The figure shows three views and two pictorial views of one solid part (mm, origin at its lowest corner). Answer the questions. A direction names the side the tool comes from. Round coordinates to 2 decimals unless told otherwise and drop trailing zeros. Order: outer loops, then holes, each group sorted by start corner. A loop starts at its lowest first (then second) coordinate and runs counter-clockwise, first axis right, second up. Notation, with made-up numbers: (30.5, 62.5) -> (88.5, 62.5) arc R19 ccw to (88.5, 91.5) -> close; hole circle Ø11 at (13, -25.75). An arc over 180 degrees is marked (long way). Answer as a JSON object with one key per item and string values. Group by question number.
Item 1: Given P1, Ø4, axis at x = 33.5, y = 25, coming from the +Z side; P2, Ø1, axis at x = 17, y = 8, coming from the -Z side; P3, Ø5.5, axis at x = 11.5, y = 24, coming from the +Z side (1 decimal), each flat-ended and moving along its own axis, determine where each tip first touches the part or whether it passes through.
Item 2: The mould has two halves that part along Z. Classify the marked faces 4, 5, 6 and 7: pulls with the +Z half, pulls with the -Z half, needs draft (parallel to the pull), parting line crosses it, or undercut.
Item 3: Section C-C, the plane y = 22.5 is taken. Write down the section's boundary in (x, z).
Item 4: Section A-A, the plane z = 6 is taken. Write down the section's boundary in (x, y).
Item 5: Consider probe 1 along X at (y, z) = (11, 5.5); probe 2 along Z at (x, y) = (12, 26); probe 3 along Z at (x, y) = (32, 26.5). Determine where each line is inside the solid, lowest interval first. Write a range as from..to.
Item 6: For the marked faces 1, 2 and 3, determine the directions among +Z, -Z, +X, -X, +Y, -Y from which every point of the face is accessible in a straight line to the end or side of a thin tool.
Item 7: Section B-B, the plane x = 12.5 is taken. Write down the section's boundary in (y, z).
Item 8: Section D-D, the plane z = 19 is taken. Write down the section's boundary in (x, y).
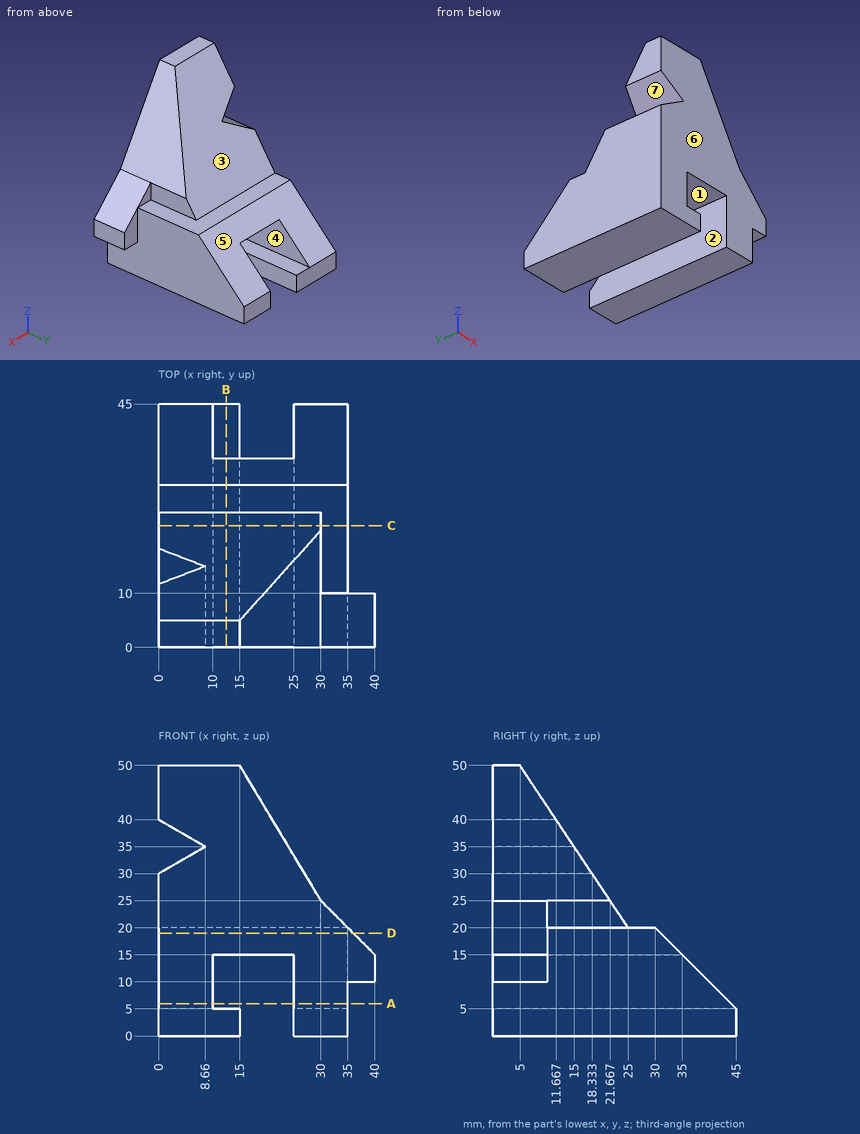
Values found:
{
 "1": {"P1": "z = 20", "P2": "z = 15", "P3": "z = 25.6"},
 "2": {"face 4": "undercut", "face 5": "pulls with the +Z half", "face 6": "needs draft", "face 7": "undercut"},
 "3": {"outline": "(0, 0) -> (15, 0) -> (15, 5) -> (10, 5) -> (10, 15) -> (25, 15) -> (25, 0) -> (35, 0) -> (35, 20) -> (30, 20) -> (30, 23.75) -> (0, 23.75) -> close"},
 "4": {"outline": "(0, 0) -> (10, 0) -> (10, 44) -> (0, 44) -> close; (25, 0) -> (35, 0) -> (35, 44) -> (25, 44) -> close"},
 "5": {"probe 1": "0..10, 25..35", "probe 2": "0..5, 15..20", "probe 3": "0..20"},
 "6": {"face 1": "+Y, -Y", "face 2": "-Z, +Y, -Y", "face 3": "+Z, +X, -X, +Y"},
 "7": {"outline": "(0, 0) -> (45, 0) -> (45, 5) -> (0, 5) -> close; (0, 15) -> (35, 15) -> (30, 20) -> (25, 20) -> (5, 50) -> (0, 50) -> close"},
 "8": {"outline": "(0, 0) -> (36, 0) -> (36, 10) -> (35, 10) -> (35, 31) -> (0, 31) -> close"}
}
